```python
from build123d import *

# Parameters (mm, degrees)
SKETCH2_W           = 12.3
SKETCH2_H           = 25.6
BOSS_EXTRUDE2_DEPTH = 3.5
SKETCH3_R           = 1
SKETCH3_W           = 5.3
SKETCH3_H           = 6.5
CUT_EXTRUDE1_DEPTH  = 3.5
FILLET1_R           = 1
FILLET2_R           = 6
SKETCH4_R           = 5.2
SKETCH4_R_2         = 3.5
BOSS_EXTRUDE3_DEPTH = 2.5


with BuildPart() as part:
    # Sketch2 → Boss-Extrude2 (new body)
    with BuildSketch(Plane.XY.offset(8)):
        with Locations((-295.104618969, 227.705749953)):
            Rectangle(SKETCH2_W, SKETCH2_H)
    extrude(amount=BOSS_EXTRUDE2_DEPTH)

    # Sketch3 → Cut-Extrude1 (cut)
    with BuildSketch(Plane.XY.offset(11.5)):
        with Locations((-299.082028179, 237.944260964)):
            Circle(SKETCH3_R)
        with Locations((-291.082028179, 237.944260964)):
            Circle(SKETCH3_R)
        with Locations((-294.942907715, 231.542892456)):
            Rectangle(SKETCH3_W, SKETCH3_H)
    extrude(amount=-CUT_EXTRUDE1_DEPTH, mode=Mode.SUBTRACT)

    # Fillet1
    fillet1_edges = [part.edges().sort_by_distance(p)[0] for p in [
        (-297.592907715, 228.292892456, 9.75),
        (-297.592907715, 234.792892456, 9.75),
        (-292.292907715, 234.792892456, 9.75),
        (-292.292907715, 228.292892456, 9.75),
        (-301.254618969, 240.505749953, 9.75),
        (-288.954618969, 240.505749953, 9.75),
    ]]
    fillet(fillet1_edges, radius=FILLET1_R)

    # Fillet2
    fillet2_edges = [part.edges().sort_by_distance(p)[0] for p in [
        (-288.954618969, 214.905749953, 9.75),
        (-301.254618969, 214.905749953, 9.75),
    ]]
    fillet(fillet2_edges, radius=FILLET2_R)

    # Sketch4 → Boss-Extrude3 (add)
    with BuildSketch(Plane.XY.offset(11.5)):
        with Locations((-295.004474021, 220.905749953)):
            Circle(SKETCH4_R)
        with Locations((-295.004474021, 220.905749953)):
            Circle(SKETCH4_R_2, mode=Mode.SUBTRACT)
    extrude(amount=BOSS_EXTRUDE3_DEPTH)


solid = part.part
```
Read the model definition and answer for the solid it produces. Units are mm, in the model's axes. A direction names the side the tool comes from. Coordinates: 2 decimals unless noted, no trailing zeros. Loops run counter-clockwise (first coordinate to the right, second up) from the corner with the lowest first, then second, coordinate; pieces in that order, holes last.
(1) The mould has two halves that part along X. Classify faces 4 (the face through (-297.3, 234.5, 9.7)), 5 (the face through (-296.13, 215.83, 12.73)), 6 (the face through (-301.255, 230, 10)), 7 (the face through (-297.292, 228.578, 9.726)): released by +X, released by -X, zero draft, split by the parting line, or undercut.
Solution:
face 4: undercut
face 5: split by the parting line
face 6: released by -X
face 7: undercut
(2) The part is cut by section D-D (z = 11). Determine the outline of the cut face in (x, y), and give its area (3 significant figures).
Solution:
outline: (-301.25, 220.91) arc R6 ccw to (-295.25, 214.91) - (-294.95, 214.91) arc R6 ccw to (-288.95, 220.91) - (-288.95, 239.51) arc R1 ccw to (-289.95, 240.51) - (-300.25, 240.51) arc R1 ccw to (-301.25, 239.51) - close; hole circle Ø2 at (-299.08, 237.94); hole (-297.59, 229.29) arc R1 ccw to (-296.59, 228.29) - (-293.29, 228.29) arc R1 ccw to (-292.29, 229.29) - (-292.29, 233.79) arc R1 ccw to (-293.29, 234.79) - (-296.59, 234.79) arc R1 ccw to (-297.59, 233.79) - close; hole circle Ø2 at (-291.08, 237.94)
area: 259 mm2
(3) The part is cut by section C-C (z = 12.2). Determine the outline of the cut face in (x, y), and give its area (3 significant figures).
Solution:
outline: circle Ø10.4 at (-295, 220.91); hole circle Ø7 at (-295, 220.91)
area: 46.5 mm2
(4) A tool of negligible diameter and unlimited length cuts with its end or side. For faces 1 (the face through (-293.39, 217.8, 12.73)), 2 (the face through (-292.59, 228.58, 9.73)), 3 (the face through (-289.255, 240.221, 9.774)), from which of +Z, -Z, +X, -X, +Y, -Y can it reach the whole face along a straight path? Write none if from no direction.
Solution:
face 1: +Z
face 2: +Z, -Z
face 3: +Z, -Z, +X, +Y
(5) Flat-ended cylindrical pins translate along their axes: pin 1 Ø2.5 at (x, y) = (-299.08, 237.94) entering from +Z; pin 2 Ø1 at (x, z) = (-292, 11.5) entering from -Y. Find the tip coordinate at first contact, or state that the pin passes through.
Solution:
pin 1: stops at z = 11.5
pin 2: stops at y = 215.43
(6) The part is cut by section A-A (x = -293). Determine the outline of the cut face in (y, z), and give its area (3 significant figures).
Solution:
outline: (215.23, 8) - (228.34, 8) - (228.34, 11.5) - (225.7, 11.5) - (225.7, 14) - (223.77, 14) - (223.77, 11.5) - (218.04, 11.5) - (218.04, 14) - (216.11, 14) - (216.11, 11.5) - (215.23, 11.5) - close; (234.75, 8) - (240.51, 8) - (240.51, 11.5) - (234.75, 11.5) - close
area: 75.7 mm2
(7) Consider line 1 along X through (y, z) = (230.75, 9.2); line 2 along Y through (x, z) = (-294.75, 9.55); line 3 along Z through (x, y) = (-294.5, 217.75). Determine where each line is inside the solid, lowest interval first.
Solution:
line 1: x = -301.25 to -297.59, -292.29 to -288.95
line 2: y = 214.91 to 228.29, 234.79 to 240.51
line 3: z = 8 to 11.5
(8) The part is cut by section B-B (y = 221.5). Determine the outline of the cut face in (x, z), and give its area (3 significant figures).
Solution:
outline: (-301.25, 8) - (-288.95, 8) - (-288.95, 11.5) - (-289.84, 11.5) - (-289.84, 14) - (-291.56, 14) - (-291.56, 11.5) - (-298.45, 11.5) - (-298.45, 14) - (-300.17, 14) - (-300.17, 11.5) - (-301.25, 11.5) - close
area: 51.6 mm2
